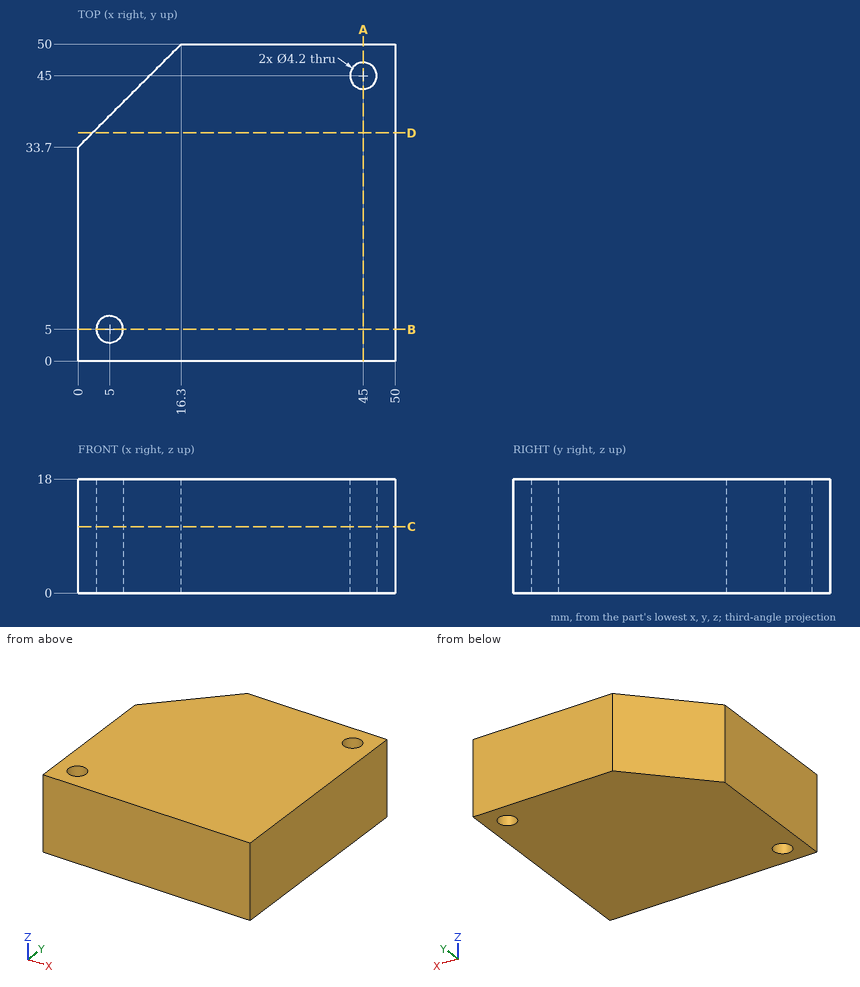
Answer from the drawing. Dimensions are ordinates in mm from the lowest x, y and z of the part. Coordinates: 2 decimals unless noted, no trailing zeros. Loops run counter-clockwise (first coordinate to the right, second up) from the corner with the lowest first, then second, coordinate; pieces in that order, holes last. Notation, with made-up numbers: (78.25, 38) - (128.25, 38) arc R18 cw to (128.25, 61) - close; hole circle Ø4 at (39, 52.5). An arc over 180 degrees is marked (long way). Answer in a Markdown table with one row per item.
1. Find section A-A, the plane x = 45. Write down the section's boundary in (y, z).
Conclusion:
| item | result |
|---|---|
| outline | (0, 0) - (42.9, 0) - (42.9, 18) - (0, 18) - close; (47.1, 0) - (50, 0) - (50, 18) - (47.1, 18) - close |
2. Straight lines are drawn through the part: line 1 (Y direction, x = 45, z = 12.5); line 2 (Y direction, x = 5, z = 11.75); line 3 (Y direction, x = 13.5, z = 2.75). For each, find the intervals that lie inside material, in ascending order.
Conclusion:
| item | result |
|---|---|
| line 1 | y = 0 to 42.9, 47.1 to 50 |
| line 2 | y = 0 to 2.9, 7.1 to 38.7 |
| line 3 | y = 0 to 47.2 |
3. Find section D-D, the plane y = 36. Write down the section's boundary in (x, z).
Conclusion:
| item | result |
|---|---|
| outline | (2.3, 0) - (50, 0) - (50, 18) - (2.3, 18) - close |
4. Find section B-B, the plane y = 5. Write down the section's boundary in (x, z).
Conclusion:
| item | result |
|---|---|
| outline | (0, 0) - (2.9, 0) - (2.9, 18) - (0, 18) - close; (7.1, 0) - (50, 0) - (50, 18) - (7.1, 18) - close |
5. Find section C-C, the plane z = 10.5. Write down the section's boundary in (x, y), then the cut area to 3 significant figures.
Conclusion:
| item | result |
|---|---|
| outline | (0, 0) - (50, 0) - (50, 50) - (16.3, 50) - (0, 33.7) - close; hole circle Ø4.2 at (5, 5); hole circle Ø4.2 at (45, 45) |
| area | 2,340 mm² |
